The figure shows three views and two pictorial views of one solid part (mm, origin at its lowest corner). Answer the questions. A direction names the side the tool comes from. Coordinates: 2 decimals unless noted, no trailing zeros. Write each loop counter-clockwise with the first axis right and the second up, starting at its lowest first coordinate (ties: lowest second). Pieces come first, ordered by that corner, then holes.
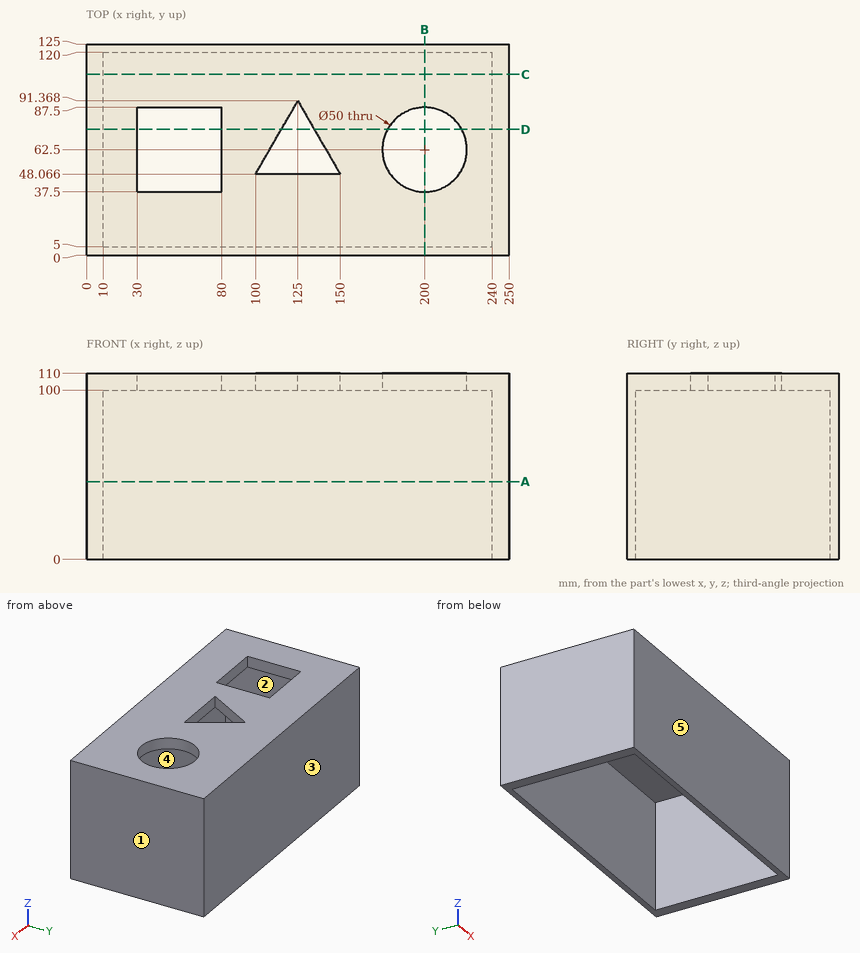
Q1. Determine the mould class of the marked faces 1, 2 and 3 for opening direction Y: released by +Y, released by -Y, zero draft, split by the parting line, or undercut.
Answers below:
face 1: zero draft
face 2: undercut
face 3: released by +Y
Q2. The part is cut by section D-D, the plane y = 74.5. Write down the section's boundary in (x, z), then the cut area to 3 significant figures.
Answers below:
outline: (0, 0) - (10, 0) - (10, 100) - (30, 100) - (30, 110) - (0, 110) - close; (80, 100) - (115.26, 100) - (115.26, 110) - (80, 110) - close; (134.74, 100) - (178.07, 100) - (178.07, 110) - (134.74, 110) - close; (221.93, 100) - (240, 100) - (240, 0) - (250, 0) - (250, 110) - (221.93, 110) - close
area: 3,370 mm2
Q3. The part is cut by section C-C, the plane y = 107. Write down the section's boundary in (x, z).
Answers below:
outline: (0, 0) - (10, 0) - (10, 100) - (240, 100) - (240, 0) - (250, 0) - (250, 110) - (0, 110) - close
Q4. The part is cut by section B-B, the plane x = 200. Write down the section's boundary in (y, z).
Answers below:
outline: (0, 0) - (5, 0) - (5, 100) - (37.5, 100) - (37.5, 110) - (0, 110) - close; (87.5, 100) - (120, 100) - (120, 0) - (125, 0) - (125, 110) - (87.5, 110) - close
Q5. Given pin 1 (8 mm diameter, centred on x = 215.5, y = 71.5, fed in from -Z); pin 2 (1.5 mm diameter, centred on x = 88.5, y = 52, fed in from -Z), each flat-ended and moving along its own axis, determine where each tip first touches the part or whether it passes through.
Answers below:
pin 1: passes through
pin 2: stops at z = 100
Q6. The part is cut by section A-A, the plane z = 46. Write down the section's boundary in (x, y).
Answers below:
outline: (0, 0) - (250, 0) - (250, 125) - (0, 125) - close; hole (10, 5) - (240, 5) - (240, 120) - (10, 120) - close
Q7. Find the intervals of material crossed by probe 1 along Y at (x, z) = (81, 96); probe 2 along X at (y, z) = (65.5, 41.5); probe 3 along Y at (x, z) = (200, 108.25), in increasing order.
Answers below:
probe 1: y = 0 to 5, 120 to 125
probe 2: x = 0 to 10, 240 to 250
probe 3: y = 0 to 37.5, 87.5 to 125
Q8. Which of the six approach directions +Z, -Z, +X, -X, +Y, -Y give full straight-line access (tool end or side, diameter ignored) to the marked faces 4 and 5?
Answers below:
face 4: -Z
face 5: +Z, -Z, +X, -X, -Y
